CAD build for the part. Positions are in the model's coordinates, mm. Face numbers are marked on the shaded views. A direction names the side the tool comes from. Give positions to 0.01 mm unless a question says otherwise; leave off trailing zeros. Loops run counter-clockwise (first coordinate to the right, second up) from the corner with the lowest first, then second, coordinate; pieces in that order, holes last. Notation, with made-up numbers: M 10,37.5 L 24,37.5 A23 ccw 24,71.5 Z; hole C 53.25,5 d8. An arc over 180 degrees is marked long. Answer as CSV lines item,"result".
Autodesk Inventor part; units mm, degrees
ref_plane "YZ Plane" through (0, 0, 0) normal (1, 0, 0) x (0, 1, 0)
ref_plane "XZ Plane" through (0, 0, 0) normal (0, 1, 0) x (-1, 0, 0)
ref_plane "XY Plane" through (0, 0, 0) normal (0, 0, 1) x (1, 0, 0)
sketch "Sketch1" plane through (0, 0, 0) normal (0, 0, 1) x (1, 0, 0)
  line L0 (-12.1708, 16.0073) -> (13.2292, 16.0073)
  line L1 (13.2292, 16.0073) -> (13.2292, -34.7927)
  line L2 (13.2292, -34.7927) -> (-12.1708, -34.7927)
  line L3 (-12.1708, -34.7927) -> (-12.1708, 16.0073)
  line L4 (11.9592, 14.7373) -> (-10.9008, 14.7373)
  line L5 (-10.9008, 14.7373) -> (-10.9008, -33.5227)
  line L6 (-10.9008, -33.5227) -> (11.9592, -33.5227)
  line L7 (11.9592, -33.5227) -> (11.9592, 14.7373)
  point P0 (0, 0)
  dimension "d0" = 25.4
  dimension "d1" = 50.8
  dimension "d2" = 1.27
extrude "Extrusion1" add sketch "Sketch1" along normal blind 101.6
sketch "Sketch2" plane through (-12.1708, 16.0073, 0) normal (0, 1, 0) x (1, 0, 0)
  circle A0 centre (12.7, -12.7) radius 1.7272
  line L0 (25.4, 0) -> (0, 0)
  line L1 (0, 0) -> (0, -101.6)
  point P0 (12.1708, 0)
  dimension "d5" = 3.4544
  dimension "d6" = 12.7
  dimension "d7" = 12.7
extrude "Extrusion2" cut sketch "Sketch2" against normal through all
pattern_linear "Rectangular Pattern1" count 10 spacing 25.4 along (0, 0, 1) of "Extrusion2"
sketch "Sketch4" plane through (13.2292, -34.7927, 0) normal (1, 0, 0) x (0, 0, -1)
  circle A0 centre (-76.2, 25.4) radius 14.2875
  line L0 (-101.6, 0) -> (-101.6, 50.8)
  point P0 (0, 34.7927)
  dimension "d19" = 28.575
  dimension "d20" = 25.4
extrude "Extrusion4" cut sketch "Sketch4" against normal through all
equation "\"d3\" = d13"
equation "\"d10\" = d14"
equation "\"d13\" = 101.6"
equation "\"d14\" = d13"
properties part number "Elevator VersaframeBacktrack"
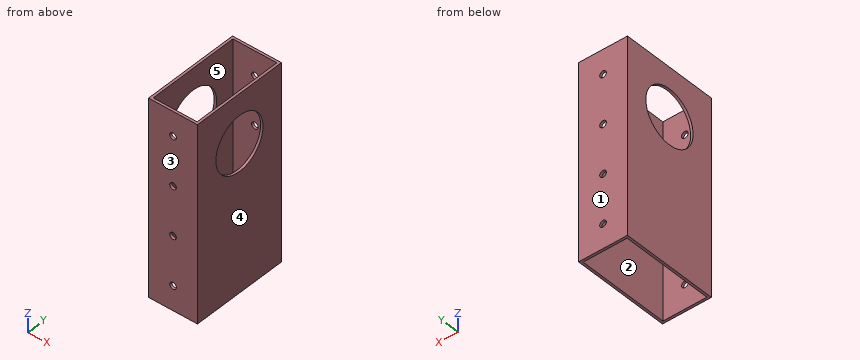
1) Drill centre lines: line 1 (Y direction, x = -4.25, z = 38.5); line 2 (X direction, y = 15, z = 38); line 3 (X direction, y = 10, z = 15). Where is each one in solid material? Low to high. Write a range as from..to.
Answer below:
line 1,"y = -34.79..-33.52, 14.74..16.01"
line 2,"x = -12.17..-1.2, 2.25..13.23"
line 3,"x = -12.17..-10.9, 11.96..13.23"
2) Band-saw the part on C-C on z = 12.7. Give the cut face in (x, y).
Answer below:
outline,"M -12.17,-34.79 L -1.2,-34.79 L -1.2,-33.52 L -10.9,-33.52 L -10.9,14.74 L -1.2,14.74 L -1.2,16.01 L -12.17,16.01 Z; M 2.26,-34.79 L 13.23,-34.79 L 13.23,16.01 L 2.26,16.01 L 2.26,14.74 L 11.96,14.74 L 11.96,-33.52 L 2.26,-33.52 Z"
3) Mould opens along Y. For the marked faces 3, 4 and 5 say: +Y half, -Y half, draft (parallel to the pull), parting line (faces both ways), or undercut.
Answer below:
face 3,"-Y half"
face 4,"draft"
face 5,"undercut"
4) Which spindle directions (+Z, -Z, +X, -X, +Y, -Y) get a long thin tool onto all of the face, cutting with end or side? Do the marked faces 1 and 2. Say none if no direction does.
Answer below:
face 1,"+Z, -Z, +X, -X, +Y"
face 2,"+Z, -Z"
5) Band-saw the part on A-A on y = -28. Give the cut face in (x, z).
Answer below:
outline,"M -12.17,0 L -10.9,0 L -10.9,101.6 L -12.17,101.6 Z; M 11.96,0 L 13.23,0 L 13.23,101.6 L 11.96,101.6 Z"
6) Band-saw the part on B-B on x = -9.75. Give the cut face in (y, z).
Answer below:
outline,"M -34.79,0 L -33.52,0 L -33.52,101.6 L -34.79,101.6 Z; M 14.74,0 L 16.01,0 L 16.01,101.6 L 14.74,101.6 Z"
7) Flat gauge pins, fed straight in: pin 1 (3 mm diameter, centred on x = 0.53, z = 88.9, fed in from -Y); pin 2 (6 mm diameter, centred on y = -20.5, z = 81.5, fed in from +X). Where does each tip first touch, or does it go through?
Answer below:
pin 1,"passes through"
pin 2,"stops at x = 13.23"
8) Band-saw the part on D-D on z = 49.5. Give the cut face in (x, y).
Answer below:
outline,"M -12.17,-34.79 L 13.23,-34.79 L 13.23,16.01 L -12.17,16.01 Z; hole M -10.9,-33.52 L 11.96,-33.52 L 11.96,14.74 L -10.9,14.74 Z"
